Geometry check sheet. Reference: the model listing, model coordinates, mm. A direction names the side the tool comes from. Coordinates: 2 decimals unless noted, no trailing zeros. Loops run counter-clockwise (first coordinate to the right, second up) from the corner with the lowest first, then second, coordinate; pieces in that order, holes last.
from build123d import *

# Parameters (mm, degrees)
F1_DEPTH = 15
F2_R     = 2
F3_R     = 2
F5_R     = 3
F5_R_2   = 1.9999997224


with BuildPart() as f1:
    # F0 (on Front) → F1 (new body, symmetric)
    with BuildSketch(Plane.XZ):
        Polygon((-3, 15), (-3, 30), (3, 30), (3, 15), (18, 15), (18, 18), (6, 18), (6, 33), (-6, 33), (-6, 15), align=None)
    extrude(amount=F1_DEPTH, both=True)

    # F2
    f2_edges = [f1.edges().sort_by_distance(p)[0] for p in [
        (6, 0, 33),
    ]]
    fillet(f2_edges, radius=F2_R)

    # F3
    f3_edges = [f1.edges().sort_by_distance(p)[0] for p in [
        (-6, 0, 33),
    ]]
    fillet(f3_edges, radius=F3_R)

    # F6: sweep along a path in F4
    with BuildLine(Plane.XZ) as f6_path:
        Line((-10, 0), (-10, 33))
        ThreePointArc((-10, 33), (0, 43), (10, 33))
        Line((10, 33), (10, 3))
    # F5 (on Top) → F6 (sweep)
    with BuildSketch(Plane.XY):
        with Locations((-10, 0)):
            Circle(F5_R)
        with Locations((-10, 0)):
            Circle(F5_R_2, mode=Mode.SUBTRACT)
    sweep(path=f6_path.line)


solid = f1.part
(1) Scan lines: L1, parallel to Y at x = 10, z = 21; L2, parallel to X at y = 10.5, z = 24.5; L3, parallel to Z at x = 9, y = 5.5. Record each from-to range of solid material in increasing order.
Findings:
L1: y = -3 to -2, 2 to 3
L2: x = -6 to -3, 3 to 6
L3: z = 15 to 18
(2) Sectioned sample at C-C on z = 37.5. State how many separate pieces and enclosed holes the cut face has, and give its area (3 significant figures).
Findings:
separate pieces: 2
enclosed holes: 2
area: 35.8 mm2
(3) Gauge pin test, flat ends, axial feed: pin 1 Ø4.5 at (x, y) = (10, 0) entering from -Z; pin 2 Ø4 at (x, y) = (0.5, -3) entering from +Z; pin 3 Ø5 at (x, z) = (10, 30.5) entering from -Y. Record the tip position at first contact, or that the pin passes through.
Findings:
pin 1: stops at z = 3
pin 2: stops at z = 45.82
pin 3: stops at y = -3
(4) Sectioned sample at B-B on x = 15.5. Record the cut outline in (y, z), and give its area (3 significant figures).
Findings:
outline: (-15, 15) - (15, 15) - (15, 18) - (-15, 18) - close
area: 90.0 mm2
(5) Access from +Z, -Z, +X, -X, +Y, -Y to the whole of each face (thin tool, end or side, straight path). Record for faces 1 (the flat face through (0, 0, 30)), 2 (the flat face through (8, -1, 3)), 3 (the cylindrical face through (12.4, -1.8, 8.9)), 4 (the flat face through (10, 0, 18)).
Findings:
face 1: -Z, +Y, -Y
face 2: -Z, +X, +Y, -Y
face 3: -Z
face 4: none
(6) Sectioned sample at A-A on y = -4.5. Record the cut outline in (x, z).
Findings:
outline: (-6, 15) - (-3, 15) - (-3, 30) - (3, 30) - (3, 15) - (18, 15) - (18, 18) - (6, 18) - (6, 31) arc R2 ccw to (4, 33) - (-4, 33) arc R2 ccw to (-6, 31) - close
(7) Draft check along Z on faces 5 (the flat face through (-8, -1, 0)), 6 (the flat face through (-3, 0, 22)), 7 (the cylindrical face through (12.4, -1.8, 25.4)). Enter one of: +Z half, -Z half, draft (parallel to the pull), parting line (faces both ways), or undercut.
Findings:
face 5: -Z half
face 6: draft
face 7: undercut
